Design review of the part shown in the three views and the two pictorial views. Dimensions are in mm from the part's minimum x, y and z. A direction names the side the tool comes from. Round coordinates to 2 decimals unless told otherwise and drop trailing zeros. Write each loop counter-clockwise with the first axis right and the second up, starting at its lowest first coordinate (ties: lowest second). Pieces come first, ordered by that corner, then holes. Notation, with made-up numbers: (44, 21.25) -> (60, 21.25) arc R15 ccw to (60, 30.25) -> close; hole circle Ø3 at (69.5, -30). An arc over 180 degrees is marked (long way). Answer as a JSON object with one key per item and string values. Group by question number.
1) Machinability: for the marked faces 1 and 2, which of the approach directions +Z, -Z, +X, -X, +Y, -Y give a long, thin tool a straight path to every point of the face, cutting with its end or side? Answer none if there is none.
2) We need section B-B, the plane y = 8.5. Write out the cut boundary in (x, z).
3) We need section A-A, the plane z = 4. Write out the cut boundary in (x, y).
4) To check wall thickness, follow probe 1 along X at (y, z) = (5, 3); probe 2 along Z at (x, y) = (57.5, 29.5); probe 3 along Y at (x, z) = (75, 9.5). State the ranges of each line that lie inside material, in increasing order. Write a range as [from, to].
5) Insertion check: pin 1 Ø5 at (y, z) = (23.5, 4) entering from -X; pin 2 Ø21 at (x, y) = (52.5, 38) entering from +Z; pin 3 Ø1.5 at (x, z) = (50, 7) entering from -Y; pin 4 Ø4 at (x, y) = (61, 63.5) entering from -Z. Each pin has a flat end and moves straight along its axis. Give the tip position at first contact, or say it passes through.
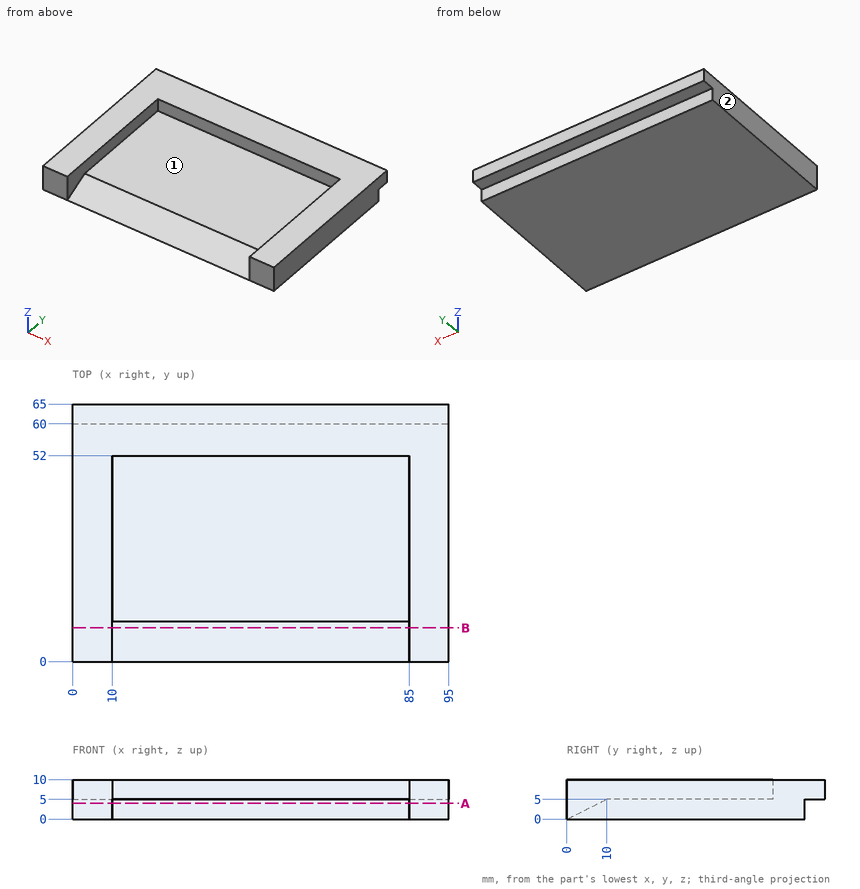
Here are the results:
{
 "1": {"face 1": "+Z, -Y", "face 2": "+Z, -Z, -X, +Y, -Y"},
 "2": {"outline": "(0, 0) -> (95, 0) -> (95, 10) -> (85, 10) -> (85, 4.25) -> (10, 4.25) -> (10, 10) -> (0, 10) -> close"},
 "3": {"outline": "(0, 0) -> (10, 0) -> (10, 8) -> (85, 8) -> (85, 0) -> (95, 0) -> (95, 60) -> (0, 60) -> close"},
 "4": {"probe 1": "x = [0, 10], [85, 95]", "probe 2": "z = [0, 5]", "probe 3": "y = [52, 65]"},
 "5": {"pin 1": "stops at x = 0", "pin 2": "stops at z = 5", "pin 3": "stops at y = 52", "pin 4": "stops at z = 5"}
}
